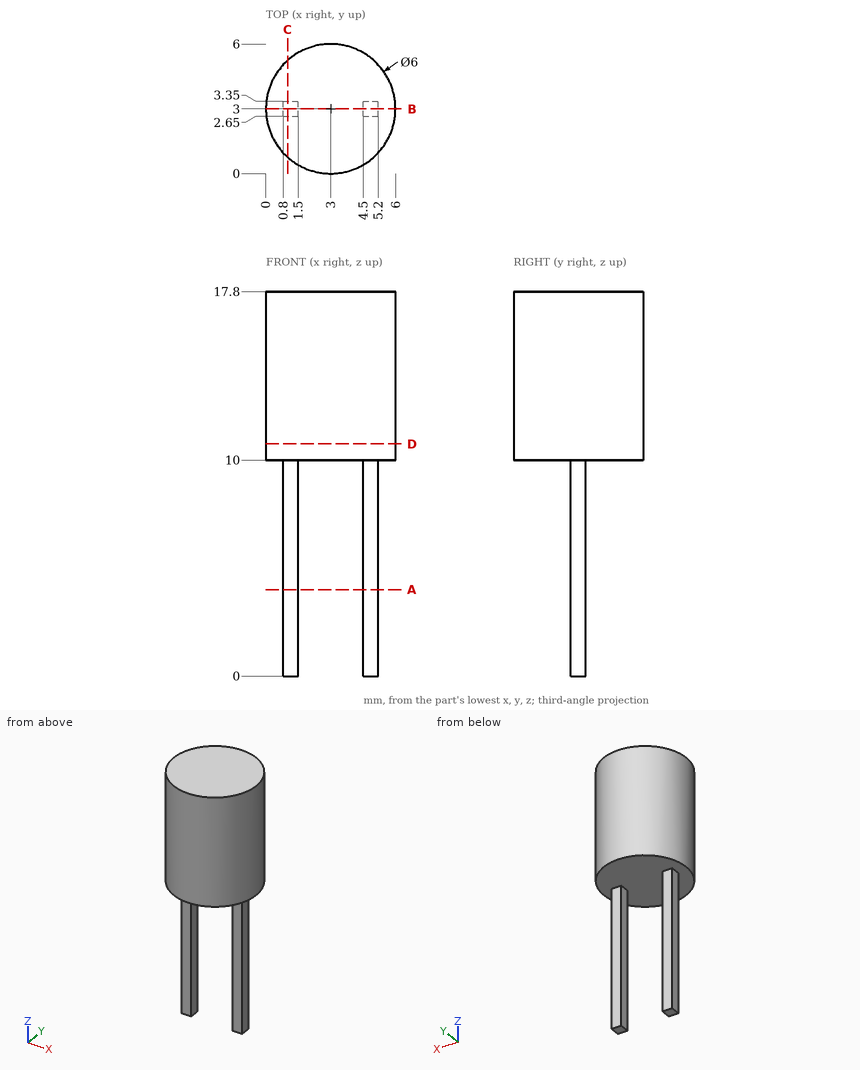
Geometry check sheet. Reference: drawing and pictorial views, mm from the part's lowest x, y, z. Round coordinates to 2 decimals unless told otherwise and drop trailing zeros. Order: outer loops, then holes, each group sorted by start corner. A loop starts at its lowest first (then second) coordinate and runs counter-clockwise, first axis right, second up. Notation, with made-up numbers: (4, -20.75) -> (15, -20.75) arc R5 cw to (15, -15.75) -> close; hole circle Ø9 at (-34.5, 23.25). An arc over 180 degrees is marked (long way). One line per item, written item: value. Start each with the question number.
Q1. Cross-section at A-A (z = 4). Record the boundary of the cut face in (x, y), and give its area (3 significant figures).
Q2. Cross-section at C-C (x = 1). Record the boundary of the cut face in (y, z), and give its area (3 significant figures).
Q3. Thickness scan on line 1 (X direction, y = 3.1, z = 16.5); line 2 (Z direction, x = 5.7, y = 3.25); line 3 (X direction, y = 2.7, z = 4). Record the ranges inside material, lowest first.
Q4. Cross-section at D-D (z = 10.75). Record the boundary of the cut face in (x, y).
Q5. Gauge pin test, flat ends, axial feed: pin 1 Ø0.6 at (x, z) = (5, 7.5) entering from -Y; pin 2 Ø0.6 at (x, z) = (5, 5) entering from +Y; pin 3 Ø0.6 at (y, z) = (3, 3) entering from -X. Record the tip position at first contact, or that the pin passes through.
Q6. Cross-section at B-B (y = 3). Record the boundary of the cut face in (x, z), and give its area (3 significant figures).
Completed:
1. outline: (0.8, 2.65) -> (1.5, 2.65) -> (1.5, 3.35) -> (0.8, 3.35) -> close; (4.5, 2.65) -> (5.2, 2.65) -> (5.2, 3.35) -> (4.5, 3.35) -> close
1. area: 0.980 mm²
2. outline: (0.76, 10) -> (2.65, 10) -> (2.65, 0) -> (3.35, 0) -> (3.35, 10) -> (5.24, 10) -> (5.24, 17.8) -> (0.76, 17.8) -> close
2. area: 41.9 mm²
3. line 1: x = 0 to 6
3. line 2: z = 10 to 17.8
3. line 3: x = 0.8 to 1.5, 4.5 to 5.2
4. outline: circle Ø6 at (3, 3)
5. pin 1: stops at y = 2.65
5. pin 2: stops at y = 3.35
5. pin 3: stops at x = 0.8
6. outline: (0, 10) -> (0.8, 10) -> (0.8, 0) -> (1.5, 0) -> (1.5, 10) -> (4.5, 10) -> (4.5, 0) -> (5.2, 0) -> (5.2, 10) -> (6, 10) -> (6, 17.8) -> (0, 17.8) -> close
6. area: 60.8 mm²
